from build123d import *

# Parameters (mm, degrees)
SKETCH1_R           = 15.494
BOSS_EXTRUDE1_DEPTH = 6.604
SKETCH2_R           = 16.764
BOSS_EXTRUDE2_DEPTH = 25.4
BOSS_EXTRUDE3_DEPTH = 7.62
FILLET1_R           = 2.54
SKETCH5_W           = 117.797362922
SKETCH5_H           = 5.08
CUT_EXTRUDE1_DEPTH  = 25.4
CUT_EXTRUDE2_DEPTH  = 25.4


with BuildPart() as part:
    # Sketch1 → Boss-Extrude1 (new body)
    with BuildSketch(Plane(origin=(0, 0, 0), x_dir=(1, 0, 0), z_dir=(0, 1, 0))):
        with Locations(Location((0, 0, 0), (0, 0, 90))):
            Circle(SKETCH1_R)
    extrude(amount=BOSS_EXTRUDE1_DEPTH)

    # Sketch2 → Boss-Extrude2 (add)
    with BuildSketch(Plane(origin=(0, 6.604, 0), x_dir=(1, 0, 0), z_dir=(0, 1, 0))):
        with Locations(Location((0, 0, 0), (0, 0, 270))):
            Circle(SKETCH2_R)
    extrude(amount=BOSS_EXTRUDE2_DEPTH)

    # Sketch4 → Boss-Extrude3 (add, symmetric)
    with BuildSketch(Plane.XY):
        Polygon((16.764, 32.004), (60.758090512, 108.204), (-60.758090512, 108.204), (-16.764, 32.004), align=None)
    extrude(amount=BOSS_EXTRUDE3_DEPTH, both=True)

    # Fillet1
    # the kernel refuses this fillet: 2.54 mm, written as the material it takes off along each edge
    with BuildSketch(Plane(origin=(56.358681461, 105.664, -5.08), x_dir=(0.8660254037844399, -0.49999999999999795, 0), z_dir=(0, 0, -1))) as fillet1_piece_1_section:
        Polygon((0, 0), (FILLET1_R, 0), (FILLET1_R, -FILLET1_R * 1.73205080757), (-FILLET1_R * 0.5, -FILLET1_R * 0.866025403784), align=None)
    fillet1_piece_1 = extrude(amount=FILLET1_R, mode=Mode.PRIVATE)
    fillet1_piece_1 = fillet1_piece_1 - Plane(origin=(56.358681461, 105.664, -5.08), x_dir=(-0.8660254037844382, -0.500000000000001, 0), z_dir=(0, 0, -1)) * Sphere(FILLET1_R, mode=Mode.PRIVATE)
    add(fillet1_piece_1, mode=Mode.SUBTRACT)
    with BuildSketch(Plane(origin=(-56.358681461, 105.664, -5.08), x_dir=(0, 1, 0), z_dir=(0, 0, -1))) as fillet1_piece_2_section:
        Polygon((0, 0), (FILLET1_R, 0), (FILLET1_R, -FILLET1_R * 1.73205080757), (-FILLET1_R * 0.5, -FILLET1_R * 0.866025403784), align=None)
    fillet1_piece_2 = extrude(amount=FILLET1_R, mode=Mode.PRIVATE)
    fillet1_piece_2 = fillet1_piece_2 - Plane(origin=(-56.358681461, 105.664, -5.08), x_dir=(0.8660254037844382, -0.500000000000001, 0), z_dir=(0, 0, -1)) * Sphere(FILLET1_R, mode=Mode.PRIVATE)
    add(fillet1_piece_2, mode=Mode.SUBTRACT)
    with BuildSketch(Plane(origin=(56.358681461, 105.664, 5.08), x_dir=(0.8660254037844399, -0.49999999999999795, 0), z_dir=(0, 0, 1))) as fillet1_piece_3_section:
        Polygon((0, 0), (FILLET1_R, 0), (FILLET1_R, FILLET1_R * 1.73205080757), (-FILLET1_R * 0.5, FILLET1_R * 0.866025403784), align=None)
    fillet1_piece_3 = extrude(amount=FILLET1_R, mode=Mode.PRIVATE)
    fillet1_piece_3 = fillet1_piece_3 - Plane(origin=(56.358681461, 105.664, 5.08), x_dir=(-0.8660254037844382, -0.500000000000001, 0), z_dir=(0, 0, 1)) * Sphere(FILLET1_R, mode=Mode.PRIVATE)
    add(fillet1_piece_3, mode=Mode.SUBTRACT)
    with BuildSketch(Plane(origin=(-56.358681461, 105.664, 5.08), x_dir=(-0.8660254037844399, -0.49999999999999795, 0), z_dir=(0, 0, 1))) as fillet1_piece_4_section:
        Polygon((0, 0), (FILLET1_R, 0), (FILLET1_R, -FILLET1_R * 1.73205080757), (-FILLET1_R * 0.5, -FILLET1_R * 0.866025403784), align=None)
    fillet1_piece_4 = extrude(amount=FILLET1_R, mode=Mode.PRIVATE)
    fillet1_piece_4 = fillet1_piece_4 - Plane(origin=(-56.358681461, 105.664, 5.08), x_dir=(0.8660254037844382, -0.500000000000001, 0), z_dir=(0, 0, 1)) * Sphere(FILLET1_R, mode=Mode.PRIVATE)
    add(fillet1_piece_4, mode=Mode.SUBTRACT)
    with BuildSketch(Plane(origin=(13.589, 26.504738686, -7.62), x_dir=(-0.8660254037844398, 0.499999999999998, 0), z_dir=(0.49999999999999795, 0.8660254037844399, 0))) as fillet1_piece_5_section:
        with BuildLine():
            CenterArc((FILLET1_R, FILLET1_R), FILLET1_R, 180, 90)
            Line((0, FILLET1_R), (0, 0))
            Line((0, 0), (FILLET1_R, 0))
        make_face()
    fillet1_piece_5 = extrude(amount=89.938771973, mode=Mode.PRIVATE)
    fillet1_piece_5 = split(fillet1_piece_5, bisect_by=Plane(origin=(37.078105995, 32.004, -7.046175079), z_dir=(0, 1, 0)), keep=Keep.TOP, mode=Mode.PRIVATE)
    add(fillet1_piece_5, mode=Mode.SUBTRACT)
    with BuildSketch(Plane(origin=(56.358681461, 108.204, -7.62), x_dir=(0, -1, 0), z_dir=(-1, 0, 0))) as fillet1_piece_6:
        with BuildLine():
            CenterArc((FILLET1_R, FILLET1_R), FILLET1_R, 180, 90)
            Line((0, FILLET1_R), (0, 0))
            Line((0, 0), (FILLET1_R, 0))
        make_face()
    extrude(amount=112.717362922, mode=Mode.SUBTRACT)
    with BuildSketch(Plane(origin=(60.758090512, 108.204, -5.08), x_dir=(-0.49999999999999645, -0.8660254037844407, 0), z_dir=(0, 0, 1))) as fillet1_piece_7:
        with BuildLine():
            CenterArc((FILLET1_R * 1.73205080757, -FILLET1_R), FILLET1_R, 90, 120)
            Line((FILLET1_R * 0.866025403784, -FILLET1_R * 1.5), (0, 0))
            Line((0, 0), (FILLET1_R * 1.73205080757, 0))
        make_face()
    extrude(amount=10.16, mode=Mode.SUBTRACT)
    with BuildSketch(Plane(origin=(-58.558385987, 104.394, -7.62), x_dir=(0, 0, 1), z_dir=(0.49999999999999795, -0.8660254037844399, 0))) as fillet1_piece_8_section:
        with BuildLine():
            CenterArc((FILLET1_R, -FILLET1_R), FILLET1_R, 90, 90)
            Line((0, -FILLET1_R), (0, 0))
            Line((0, 0), (FILLET1_R, 0))
        make_face()
    fillet1_piece_8 = extrude(amount=89.938771973, mode=Mode.PRIVATE)
    fillet1_piece_8 = split(fillet1_piece_8, bisect_by=Plane(origin=(-37.078105995, 32.004, -7.046175079), z_dir=(0, 1, 0)), keep=Keep.TOP, mode=Mode.PRIVATE)
    add(fillet1_piece_8, mode=Mode.SUBTRACT)
    with BuildSketch(Plane(origin=(-60.758090512, 108.204, -5.08), x_dir=(0.4999999999999989, -0.8660254037844393, 0), z_dir=(0, 0, 1))) as fillet1_piece_9:
        with BuildLine():
            CenterArc((FILLET1_R * 1.73205080757, FILLET1_R), FILLET1_R, 150, 120)
            Line((FILLET1_R * 0.866025403784, FILLET1_R * 1.5), (0, 0))
            Line((0, 0), (FILLET1_R * 1.73205080757, 0))
        make_face()
    extrude(amount=10.16, mode=Mode.SUBTRACT)
    with BuildSketch(Plane(origin=(13.589, 26.504738686, 7.62), x_dir=(-0.8660254037844398, 0.499999999999998, 0), z_dir=(0.49999999999999795, 0.8660254037844399, 0))) as fillet1_piece_10_section:
        with BuildLine():
            CenterArc((FILLET1_R, -FILLET1_R), FILLET1_R, 90, 90)
            Line((0, -FILLET1_R), (0, 0))
            Line((0, 0), (FILLET1_R, 0))
        make_face()
    fillet1_piece_10 = extrude(amount=89.938771973, mode=Mode.PRIVATE)
    fillet1_piece_10 = split(fillet1_piece_10, bisect_by=Plane(origin=(37.078105995, 32.004, 7.046175079), z_dir=(0, 1, 0)), keep=Keep.TOP, mode=Mode.PRIVATE)
    add(fillet1_piece_10, mode=Mode.SUBTRACT)
    with BuildSketch(Plane(origin=(56.358681461, 108.204, 7.62), x_dir=(0, -1, 0), z_dir=(-1, 0, 0))) as fillet1_piece_11:
        with BuildLine():
            CenterArc((FILLET1_R, -FILLET1_R), FILLET1_R, 90, 90)
            Line((0, -FILLET1_R), (0, 0))
            Line((0, 0), (FILLET1_R, 0))
        make_face()
    extrude(amount=112.717362922, mode=Mode.SUBTRACT)
    with BuildSketch(Plane(origin=(-58.558385987, 104.394, 7.62), x_dir=(0.8660254037844399, 0.499999999999998, 0), z_dir=(0.49999999999999795, -0.8660254037844399, 0))) as fillet1_piece_12_section:
        with BuildLine():
            CenterArc((FILLET1_R, -FILLET1_R), FILLET1_R, 90, 90)
            Line((0, -FILLET1_R), (0, 0))
            Line((0, 0), (FILLET1_R, 0))
        make_face()
    fillet1_piece_12 = extrude(amount=89.938771973, mode=Mode.PRIVATE)
    fillet1_piece_12 = split(fillet1_piece_12, bisect_by=Plane(origin=(-37.078105995, 32.004, 7.046175079), z_dir=(0, 1, 0)), keep=Keep.TOP, mode=Mode.PRIVATE)
    add(fillet1_piece_12, mode=Mode.SUBTRACT)

    # Sketch5 → Cut-Extrude1 (cut)
    with BuildSketch(Plane(origin=(0, 108.204, 0), x_dir=(1, 0, 0), z_dir=(0, 1, 0))):
        Rectangle(SKETCH5_W, SKETCH5_H)
    extrude(amount=-CUT_EXTRUDE1_DEPTH, mode=Mode.SUBTRACT)

    # Sketch6 → Cut-Extrude2 (cut)
    with BuildSketch(Plane(origin=(0, 0, -7.62), x_dir=(-1, 0, 0), z_dir=(0, 0, -1))):
        with BuildLine():
            Line((-40.64, 100.584), (40.64, 100.584))
            ThreePointArc((40.64, 100.584), (43.18, 98.044), (40.64, 95.504))
            Line((40.64, 95.504), (-40.64, 95.504))
            ThreePointArc((-40.64, 95.504), (-43.18, 98.044), (-40.64, 100.584))
        make_face()
    extrude(amount=-CUT_EXTRUDE2_DEPTH, mode=Mode.SUBTRACT)


solid = part.part
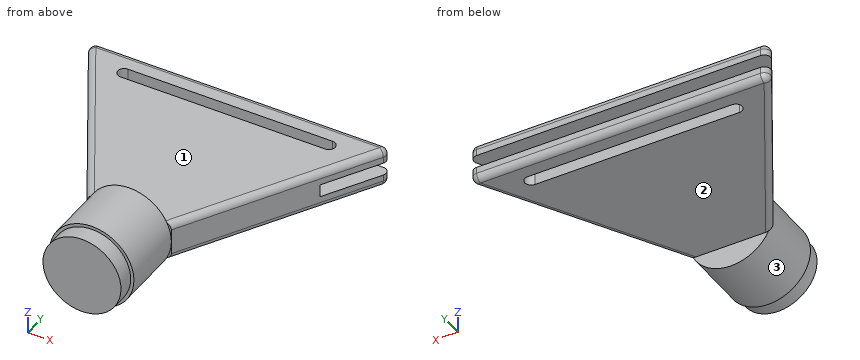
Work out the finished part from the listing and answer in its coordinate system (mm). Face numbers are marked on the shaded views. A direction names the side the tool comes from. Coordinates: 2 decimals unless noted, no trailing zeros. Write each loop counter-clockwise with the first axis right and the second up, starting at its lowest first coordinate (ties: lowest second). Pieces come first, ordered by that corner, then holes. Notation, with made-up numbers: M 66,30.25 L 74,30.25 A19 cw 74,50.25 Z; hole C 55,-17 d5. An arc over 180 degrees is marked long. Answer as CSV lines item,"result". Start each with the question number.
Item 1: Section B-B on z = -11.5 is taken. Write down the section's boundary in (x, y), and give its area (3 significant figures).
Item 2: A tool of negligible diameter and unlimited length cuts with its end or side. For the marked faces 1, 2 and 3, from which of +Z, -Z, +X, -X, +Y, -Y can it reach the whole face along a straight path? Write none if from no direction.
Item 3: Section A-A on x = 0 is taken. Write down the section's boundary in (y, z), and give its area (3 significant figures).
Item 4: Flat-ended cylindrical pins translate along their axes: P1, Ø5, axis at x = 22.5, y = 84, coming from the +Z side; P2, Ø2, axis at x = 36.5, z = 7, coming from the -Y side; P3, Ø10, axis at y = 21, z = -7, coming from the +X side; P4, Ø5, axis at x = 46, z = 11, coming from the -Y side. Find the tip coordinate at first contact, or state that the pin passes through.
Item 5: Consider L1, parallel to Z at x = -14, y = 95; L2, parallel to Y at x = -9.5, z = 10.5; L3, parallel to Z at x = 0, y = 71. Determine where each line is inside the solid, lowest interval first.
Item 6: Section D-D on y = 17 is taken. Write down the section's boundary in (x, z), and give its area (3 significant figures).
Item 7: Section C-C on x = 12.5 is taken. Write down the section's boundary in (y, z) (3 decimals).
Checks:
1,outline,"M -12.2,6.6 L -10.38,6.6 L -10.38,0 L 10.38,0 L 10.38,6.6 L 12.2,6.6 L 12.2,32 L -12.2,32 Z"
1,area,"757 mm²"
2,face 1,"+Z, +X, -X, +Y"
2,face 2,"-Z, +X, -X, +Y"
2,face 3,"-Y"
3,outline,"M 0,-15.49 L 6.6,-15.49 L 6.6,-16.76 L 32,-16.76 L 32,-7.62 L 95.5,-7.62 L 95.5,-2.54 L 82.8,-2.54 L 82.8,2.54 L 95.5,2.54 L 95.5,7.62 L 32,7.62 L 32,16.76 L 6.6,16.76 L 6.6,15.49 L 0,15.49 Z; M 100.58,-7.62 L 105.66,-7.62 A2.54 ccw 108.2,-5.08 L 108.2,-2.54 L 100.58,-2.54 Z; M 100.58,2.54 L 108.2,2.54 L 108.2,5.08 A2.54 ccw 105.66,7.62 L 100.58,7.62 Z"
3,area,"2,030 mm²"
4,P1,"stops at z = 7.62"
4,P2,"stops at y = 65.54"
4,P3,"stops at x = 16.64"
4,P4,"passes through"
5,L1,"z = -7.62 to -2.54, 2.54 to 7.62"
5,L2,"y = 0 to 32"
5,L3,"z = -7.62 to 7.62"
6,outline,"C 0,0 d33.53"
6,area,"883 mm²"
7,outline,"M 0,-9.155 L 6.604,-9.155 L 6.604,-11.171 L 32.004,-11.171 L 32.004,-7.62 L 95.504,-7.62 L 95.504,-2.54 L 82.804,-2.54 L 82.804,2.54 L 95.504,2.54 L 95.504,7.62 L 32.004,7.62 L 32.004,11.171 L 6.604,11.171 L 6.604,9.155 L 0,9.155 Z; M 100.584,-7.62 L 105.664,-7.62 A2.54 ccw 108.204,-5.08 L 108.204,-2.54 L 100.584,-2.54 Z; M 100.584,2.54 L 108.204,2.54 L 108.204,5.08 A2.54 ccw 105.664,7.62 L 100.584,7.62 Z"
